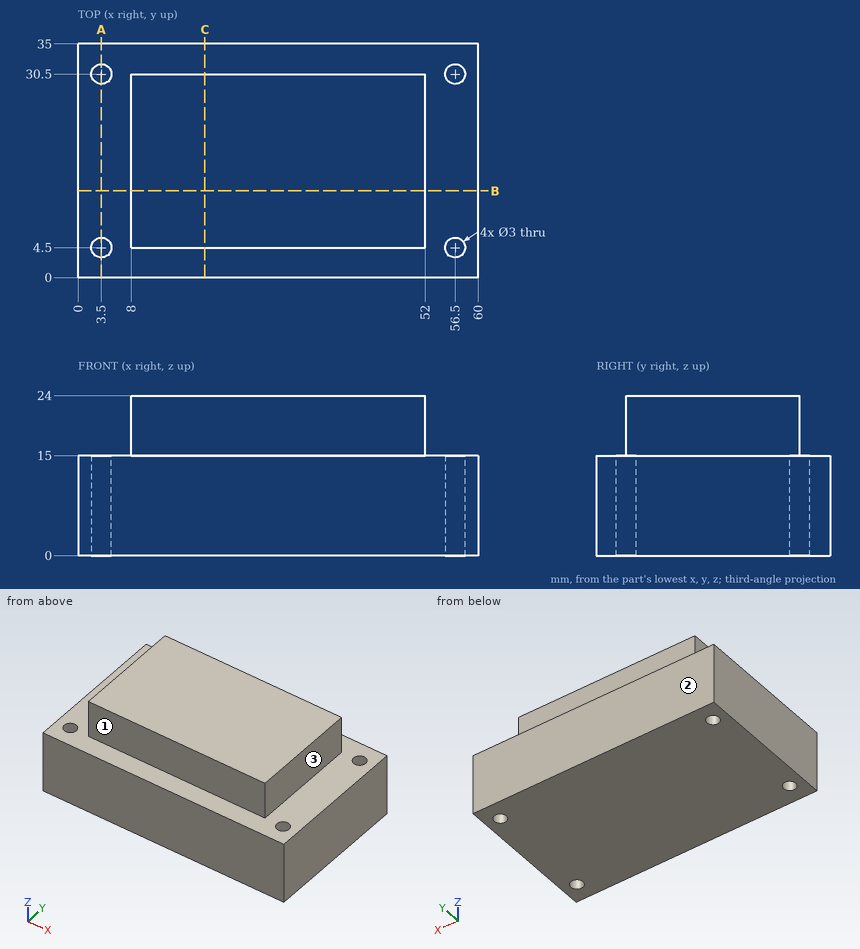
Verification items for this drawing (mm, ordinates from the low corner). A direction names the side the tool comes from. Coordinates: 2 decimals unless noted, no trailing zeros. Order: outer loops, then holes, each group sorted by start corner. A loop starts at its lowest first (then second) coordinate and runs counter-clockwise, first axis right, second up. Notation, with made-up numbers: (55.25, -38) -> (64.25, -38) arc R15 ccw to (64.25, -10) -> close; hole circle Ø8 at (22, 81). An arc over 180 degrees is marked (long way). Put each result on its own line as item: value. Start each with the question number.
1. Cross-section at C-C, the plane x = 19. Record the boundary of the cut face in (y, z).
2. Cross-section at B-B, the plane y = 13. Record the boundary of the cut face in (x, z).
3. Go/stop test with flat-tipped pins: pin 1 Ø1.5 at (x, z) = (24.5, 16.5) entering from -Y; pin 2 Ø5 at (x, y) = (3.5, 4.5) entering from +Z; pin 3 Ø7 at (x, z) = (20.5, 20) entering from +Y. Record where each tip stops, or that it passes through.
4. Cross-section at A-A, the plane x = 3.5. Record the boundary of the cut face in (y, z), then the cut area to 3 significant figures.
5. Material ranges on L1, parallel to Y at x = 3.5, z = 8.25; L2, parallel to X at y = 29.5, z = 14.75; L3, parallel to X at y = 19, z = 23.25, recorded low to high. Write a range as [from, to].
6. Access from +Z, -Z, +X, -X, +Y, -Y to the whole of each face (thin tool, end or side, straight path). Record for the marked faces 1, 2 and 3.
Computed:
1. outline: (0, 0) -> (35, 0) -> (35, 15) -> (30.5, 15) -> (30.5, 24) -> (4.5, 24) -> (4.5, 15) -> (0, 15) -> close
2. outline: (0, 0) -> (60, 0) -> (60, 15) -> (52, 15) -> (52, 24) -> (8, 24) -> (8, 15) -> (0, 15) -> close
3. pin 1: y = 4.5
3. pin 2: z = 15
3. pin 3: y = 30.5
4. outline: (0, 0) -> (3, 0) -> (3, 15) -> (0, 15) -> close; (6, 0) -> (29, 0) -> (29, 15) -> (6, 15) -> close; (32, 0) -> (35, 0) -> (35, 15) -> (32, 15) -> close
4. area: 435 mm2
5. L1: [0, 3], [6, 29], [32, 35]
5. L2: [0, 2.38], [4.62, 55.38], [57.62, 60]
5. L3: [8, 52]
6. face 1: +Z, +X, -X, -Y
6. face 2: +Z, -Z, +X, -X, +Y
6. face 3: +Z, +X, +Y, -Y
